Geometry check sheet. Reference: the model listing, model coordinates, mm. Face numbers are marked on the shaded views. A direction names the side the tool comes from. Give positions to 0.01 mm unless a question says otherwise; leave off trailing zeros. Order: outer loops, then holes, each group sorted by start corner. A loop starts at its lowest first (then second) coordinate and runs counter-clockwise, first axis right, second up. Notation, with made-up numbers: M -29,79 L 19,79 A18 ccw 19,114 Z; hole C -21,5 d3. An arc over 180 degrees is marked long. Put each result on its own line as item: value. Start each with the question number.
Q1. Go/stop test with flat-tipped pins: pin 1 (14 mm diameter, centred on x = 15.24, z = -19.05, fed in from +Y); pin 2 (19 mm diameter, centred on y = 2.5, z = 10.5, fed in from +X); pin 3 (2 mm diameter, centred on y = 3.5, z = 90.5, fed in from +X). Record where each tip stops, or that it passes through.
Q2. Section check C-C on y = -29.5. Record the cut outline in (x, z) (3 decimals), then the cut area to 3 significant figures.
Q3. Section check A-A on z = -19.05. Record the cut outline in (x, y) (3 decimals), then the cut area to 3 significant figures.
Q4. Section check B-B on x = 3. State how many separate pieces and enclosed holes the cut face has, then the cut area to 3 significant figures.
Q5. Section check D-D on y = -57. Record the cut outline in (x, z).
Q6. Mould release check, pull along Z, two halves, no side actions. Record for the marked faces 4, 5 and 6: +Z half, -Z half, draft (parallel to the pull), parting line (faces both ways), or undercut.
Q7. Material ranges on L1, parallel to Y at x = 10, z = 3.5; L2, parallel to Y at x = 28, z = -2.5; L3, parallel to X at y = 1, z = -19, recorded low to high.
Q8. Access from +Z, -Z, +X, -X, +Y, -Y to the whole of each face (thin tool, end or side, straight path). Record for the marked faces 1, 2 and 3.
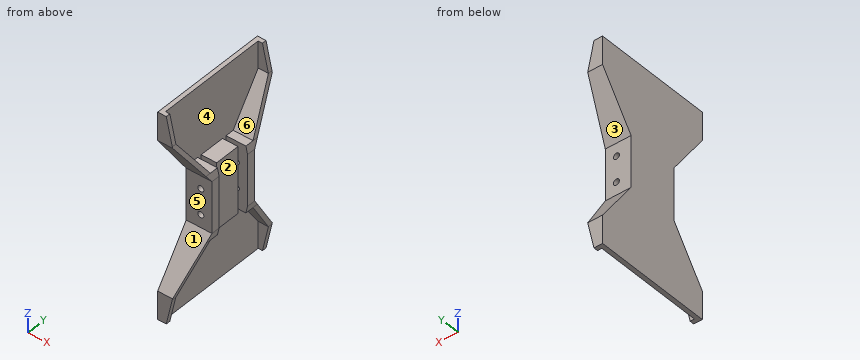
```python
from build123d import *

# Parameters (mm, degrees)
SKETCH1_W           = 19.05
SKETCH1_H           = 49.170887152
BOSS_EXTRUDE1_DEPTH = 6.35
BOSS_EXTRUDE2_START = -6.35
SKETCH1_4_W         = 19.05
SKETCH1_4_H         = 49.170887152
BOSS_EXTRUDE2_DEPTH = 38.1
CUT_EXTRUDE1_START  = 31.75
SKETCH1_6_W         = 19.05
SKETCH1_6_H         = 49.170887152
CUT_EXTRUDE1_DEPTH  = 8.89
SKETCH3_R           = 4.445
CUT_EXTRUDE2_DEPTH  = 180.268046511


with BuildPart() as part:
    # Sketch1 → Boss-Extrude1 (new body)
    with BuildSketch(Plane.YZ):
        Polygon((-19.05, 0), (-25.4, 0), (-25.4, -49.170887152), (-38.1, -49.170887152), (-82.55, -112.652066052), (-82.55, -152.4), (0, -152.4), (0, -49.170887152), (-19.05, -49.170887152), align=None)
        Polygon((-25.4, 0), (-38.1, 0), (-38.1, -38.1), (-88.9, -110.649918742), (-88.9, -152.4), (-82.55, -152.4), (-82.55, -112.652066052), (-38.1, -49.170887152), (-25.4, -49.170887152), align=None)
        with Locations((-9.525, -24.585443576)):
            Rectangle(SKETCH1_W, SKETCH1_H)
    extrude(amount=-BOSS_EXTRUDE1_DEPTH)

    # Sketch1<4> → Boss-Extrude2 (add)
    with BuildSketch(Plane.YZ.offset(BOSS_EXTRUDE2_START)):
        Polygon((-25.4, 0), (-38.1, 0), (-38.1, -38.1), (-88.9, -110.649918742), (-88.9, -152.4), (-82.55, -152.4), (-82.55, -112.652066052), (-38.1, -49.170887152), (-25.4, -49.170887152), align=None)
        with Locations((-9.525, -24.585443576)):
            Rectangle(SKETCH1_4_W, SKETCH1_4_H)
    extrude(amount=BOSS_EXTRUDE2_DEPTH)

    # Sketch1<6> → Cut-Extrude1 (cut)
    with BuildSketch(Plane.YZ.offset(CUT_EXTRUDE1_START)):
        with Locations((-9.525, -24.585443576)):
            Rectangle(SKETCH1_6_W, SKETCH1_6_H)
    extrude(amount=-CUT_EXTRUDE1_DEPTH, mode=Mode.SUBTRACT)

    # Sketch3 → Cut-Extrude2 (cut, through all)
    with BuildSketch(Plane(origin=(0, 0, 0), x_dir=(-1, 0, 0), z_dir=(0, 1, 0))):
        Polygon((-15.182874211, -112.652066052), (-29.289802855, -49.170887152), (-31.75, -49.170887152), (-31.75, -112.652066052), align=None)
        Polygon((-6.35, -152.4), (-15.182874211, -112.652066052), (-31.75, -112.652066052), (-31.75, -152.4), align=None)
        with Locations(Location((-15.24, -19.05, 0), (0, 0, 90))):
            Circle(SKETCH3_R)
        Polygon((-31.75, -38.1), (-31.75, -49.170887152), (-29.289802855, -49.170887152), align=None)
    extrude(amount=-CUT_EXTRUDE2_DEPTH, mode=Mode.SUBTRACT)

    # Mirror1: part across plane


with BuildPart() as part_1:
    add(part.part)
    add(part.part.mirror(Plane(origin=(-6.35, 0, 0), x_dir=(0, 0, 1), z_dir=(0, -1, 0))))

    # Mirror2: part across plane


with BuildPart() as part_2:
    add(part_1.part)
    add(part_1.part.mirror(Plane(origin=(-6.35, 0, 0), x_dir=(1, 0, 0), z_dir=(0, 0, 1))))


solid = part_2.part
```
Results found:
1. pin 1: stops at y = 38.1
1. pin 2: stops at x = 22.86
1. pin 3: stops at x = 0
2. outline: M -6.35,-152.4 L 0,-152.4 L 0,-49.171 L 29.29,-49.171 L 31.75,-38.1 L 31.75,38.1 L 29.29,49.171 L 0,49.171 L 0,152.4 L -6.35,152.4 Z; hole C 15.24,-19.05 d8.89; hole C 15.24,19.05 d8.89
2. area: 4,910 mm^2
3. outline: M -6.35,-38.1 L 10.795,-38.1 L 10.795,-25.4 L 0,-25.4 L 0,-19.05 L 10.795,-19.05 L 10.795,19.05 L 0,19.05 L 0,25.4 L 10.795,25.4 L 10.795,38.1 L -6.35,38.1 Z; M 19.685,-38.1 L 31.75,-38.1 L 31.75,-25.4 L 19.685,-25.4 Z; M 19.685,-19.05 L 22.86,-19.05 L 22.86,19.05 L 19.685,19.05 Z; M 19.685,25.4 L 31.75,25.4 L 31.75,38.1 L 19.685,38.1 Z
3. area: 1,600 mm^2
4. separate pieces: 3
4. enclosed holes: 0
4. area: 9,390 mm^2
5. outline: M -6.35,-152.4 L 0,-152.4 L 0,-76.16 L 23.29,-76.16 L 25.75,-65.09 L -6.35,-65.09 Z; M -6.35,65.09 L 25.75,65.09 L 23.29,76.16 L 0,76.16 L 0,152.4 L -6.35,152.4 Z
6. face 4: draft
6. face 5: undercut
6. face 6: +Z half
7. L1: y = -38.1 to -25.4, -19.05 to 19.05, 25.4 to 38.1
7. L2: y = -38.1 to -25.4, 25.4 to 38.1
7. L3: x = -6.35 to 10.8, 19.68 to 22.86
8. face 1: +X, -X, -Y
8. face 2: +Z, -Z, +X
8. face 3: +X, -X, +Y
